CAD build for the part. Positions are in the model's coordinates, mm. Give positions to 0.01 mm unless a question says otherwise; leave off trailing zeros. Write each loop counter-clockwise with the first axis right and the second up, starting at its lowest first coordinate (ties: lowest second). Pieces come first, ordered by that corner, then holes. Notation, with made-up numbers: (60, 39.5) - (84, 39.5) arc R14 cw to (84, 45.5) - close; hole circle Ø5 at (62, 51). An arc over 180 degrees is marked (long way). Put each result on its own line as item: value. Start each with the question number.
1. Mould opens along Z. For faces 1 (the flat face through (0, 19, 5)), 2 (the cylindrical face through (1.24, 18.207, -4.043)), 3 (the cylindrical face through (1.26, 8.95, 21.6)) say: +Z half, -Z half, draft (parallel to the pull), parting line (faces both ways), or undercut.
2. Cut at A-A on z = 0. List the corners of the cut face in (x, y).
3. Drop flat-ended pins along their axis: pin 1 (1.5 mm diameter, centred on x = 1.5, z = -17, fed in from -Y); pin 2 (1.5 mm diameter, centred on x = 1.5, y = 17.5, fed in from +Z). Give the stop position or say it passes through.
4. Wall check: line 1 (Y direction, x = 1.2, z = 0); line 2 (Z direction, x = 1, y = -15); line 3 (Z direction, x = 1.35, y = -8.5). Give the ranges that are in metal, low to high.
from build123d import *


with BuildPart() as part:
    # Esquisse1 → Révolution1 (revolve)
    with BuildSketch(Plane.XY, mode=Mode.PRIVATE) as r_volution1_sk:
        Polygon((0, 22.88), (0.5, 23.38), (2, 23.38), (2.5, 22.88), (2.5, 19.15), (2, 18.65), (0.5, 18.65), (0, 19.15), align=None)
    revolve(r_volution1_sk.sketch.rotate(Axis((-10.655084746, 0, 0), (1, 0, 0)), 90), axis=Axis((-10.655084746, 0, 0), (1, 0, 0)))


solid = part.part
Report:
1. face 1: draft
1. face 2: undercut
1. face 3: parting line
2. outline: (0, -22.88) - (0.5, -23.38) - (2, -23.38) - (2.5, -22.88) - (2.5, -19.15) - (2, -18.65) - (0.5, -18.65) - (0, -19.15) - close; (0, 19.15) - (0.5, 18.65) - (2, 18.65) - (2.5, 19.15) - (2.5, 22.88) - (2, 23.38) - (0.5, 23.38) - (0, 22.88) - close
3. pin 1: stops at y = -16.81
3. pin 2: stops at z = 16.31
4. line 1: y = -23.38 to -18.65, 18.65 to 23.38
4. line 2: z = -17.93 to -11.08, 11.08 to 17.93
4. line 3: z = -21.78 to -16.6, 16.6 to 21.78
